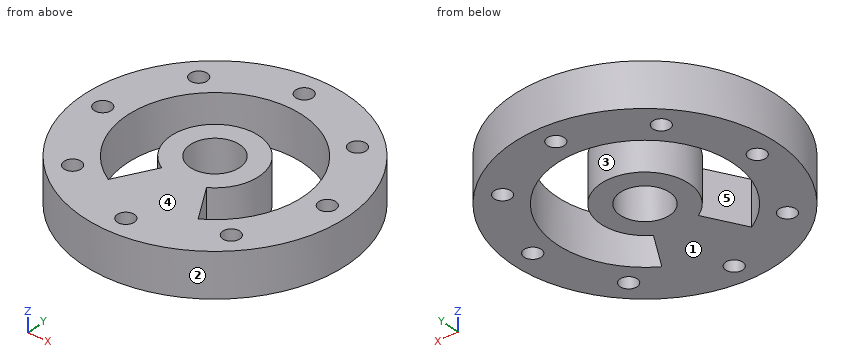
```python
from build123d import *

# Parameters (mm, degrees)
SKETCH6_R           = 24
BOSS_EXTRUDE1_DEPTH = 8
CUT_EXTRUDE4_DEPTH  = 8
SKETCH7_R           = 4.5
CUT_EXTRUDE5_DEPTH  = 8
SKETCH8_R           = 1.55
CUT_EXTRUDE6_DEPTH  = 8


with BuildPart() as part:
    # Sketch6 → Boss-Extrude1 (new body)
    with BuildSketch(Plane.XY):
        Circle(SKETCH6_R)
    extrude(amount=BOSS_EXTRUDE1_DEPTH)

    # Sketch4 → Cut-Extrude4 (cut)
    with BuildSketch(Plane.XY):
        with BuildLine():
            Line((-4, -6.92820323), (-8, -13.856406461))
            ThreePointArc((-8, -13.856406461), (0, 16), (8, -13.856406461))
            Line((8, -13.856406461), (4, -6.92820323))
            ThreePointArc((4, -6.92820323), (0, 8), (-4, -6.92820323))
        make_face()
    extrude(amount=CUT_EXTRUDE4_DEPTH, mode=Mode.SUBTRACT)

    # Sketch7 → Cut-Extrude5 (cut)
    with BuildSketch(Plane(origin=(0, 0, 0), x_dir=(-1, 0, 0), z_dir=(0, 0, -1))):
        Circle(SKETCH7_R)
    extrude(amount=-CUT_EXTRUDE5_DEPTH, mode=Mode.SUBTRACT)

    # Sketch8 → Cut-Extrude6 (cut)
    with BuildSketch(Plane(origin=(0, 0, 8), x_dir=(-1, 0, 0), z_dir=(0, 0, -1))):
        with Locations(Location((0, 20, 0), (0, 0, 180))):
            Circle(SKETCH8_R)
        with Locations(Location((14.142135624, 14.142135624, 0), (0, 0, 180))):
            Circle(SKETCH8_R)
        with Locations(Location((20, 0, 0), (0, 0, 180))):
            Circle(SKETCH8_R)
        with Locations(Location((14.142135624, -14.142135624, 0), (0, 0, 180))):
            Circle(SKETCH8_R)
        with Locations(Location((0, -20, 0), (0, 0, 180))):
            Circle(SKETCH8_R)
        with Locations(Location((-14.142135624, -14.142135624, 0), (0, 0, 180))):
            Circle(SKETCH8_R)
        with Locations(Location((-20, 0, 0), (0, 0, 180))):
            Circle(SKETCH8_R)
        with Locations(Location((-14.142135624, 14.142135624, 0), (0, 0, 180))):
            Circle(SKETCH8_R)
    extrude(amount=CUT_EXTRUDE6_DEPTH, mode=Mode.SUBTRACT)


solid = part.part
```
Geometry check sheet. Reference: the model listing, model coordinates, mm. Face numbers are marked on the shaded views. A direction names the side the tool comes from. Give positions to 0.01 mm unless a question says otherwise; leave off trailing zeros. Write each loop counter-clockwise with the first axis right and the second up, starting at its lowest first coordinate (ties: lowest second). Pieces come first, ordered by that corner, then holes.
1) Section check D-D, the plane y = -20. Record the boundary of the cut face in (x, z).
2) Section check A-A, the plane x = 0. Record the boundary of the cut face in (y, z).
3) Gauge pin test, flat ends, axial feed: pin 1 (3 mm diameter, centred on x = -1.5, z = 6.5, fed in from +Y); pin 2 (1 mm diameter, centred on y = 18.5, z = 3, fed in from +X); pin 3 (3 mm diameter, centred on y = -3.5, z = 6, fed in from +X). Record the tip position at first contact, or that the pin passes through.
4) Release check for a two-part mould opening along Y. For the marked faces 1, 2 and 3 record: pulls with the +Y half, pulls with the -Y half, needs draft (parallel to the pull), parting line crosses it, or undercut.
5) Section check B-B, the plane y = 0. Record the boundary of the cut face in (x, z).
6) Section check C-C, the plane x = -9.5. Record the boundary of the cut face in (y, z), and give its area (3 significant figures).
7) Access from +Z, -Z, +X, -X, +Y, -Y to the whole of each face (thin tool, end or side, straight path). Record for the marked faces 4 and 5.
8) Material ranges on L1, parallel to Y at x = 0, z = 4.25; L2, parallel to X at y = 14, z = 3; L3, parallel to Y at x = -2, z = 5.5, recorded low to high.
Computed:
1. outline: (-13.27, 0) - (-1.55, 0) - (-1.55, 8) - (-13.27, 8) - close; (1.55, 0) - (13.27, 0) - (13.27, 8) - (1.55, 8) - close
2. outline: (-24, 0) - (-21.55, 0) - (-21.55, 8) - (-24, 8) - close; (-18.45, 0) - (-4.5, 0) - (-4.5, 8) - (-18.45, 8) - close; (4.5, 0) - (8, 0) - (8, 8) - (4.5, 8) - close; (16, 0) - (18.45, 0) - (18.45, 8) - (16, 8) - close; (21.55, 0) - (24, 0) - (24, 8) - (21.55, 8) - close
3. pin 1: stops at y = 24
3. pin 2: stops at x = 15.87
3. pin 3: stops at x = 23.92
4. face 1: needs draft
4. face 2: parting line crosses it
4. face 3: undercut
5. outline: (-24, 0) - (-21.55, 0) - (-21.55, 8) - (-24, 8) - close; (-18.45, 0) - (-16, 0) - (-16, 8) - (-18.45, 8) - close; (-8, 0) - (-4.5, 0) - (-4.5, 8) - (-8, 8) - close; (4.5, 0) - (8, 0) - (8, 8) - (4.5, 8) - close; (16, 0) - (18.45, 0) - (18.45, 8) - (16, 8) - close; (21.55, 0) - (24, 0) - (24, 8) - (21.55, 8) - close
6. outline: (-22.04, 0) - (-12.87, 0) - (-12.87, 8) - (-22.04, 8) - close; (12.87, 0) - (22.04, 0) - (22.04, 8) - (12.87, 8) - close
6. area: 147 mm2
7. face 4: +Z, +X, -X, +Y, -Y
7. face 5: +Z, -Z
8. L1: y = -24 to -21.55, -18.45 to -4.5, 4.5 to 8, 16 to 18.45, 21.55 to 24
8. L2: x = -19.49 to -15.69, -12.6 to -7.75, 7.75 to 12.6, 15.69 to 19.49
8. L3: y = -23.92 to -4.03, 4.03 to 7.75, 15.87 to 23.92
